The model under review builds one solid part; all positions refer to its coordinate system, in mm. Face numbers are marked on the shaded views. A direction names the side the tool comes from. Coordinates: 2 decimals unless noted, no trailing zeros. Loops run counter-clockwise (first coordinate to the right, second up) from the corner with the lowest first, then second, coordinate; pieces in that order, holes last. Notation, with made-up numbers: (58, -12.5) - (116, -12.5) arc R25 ccw to (116, 10.5) - close; hole circle Ø4 at (70, 10.25). An arc over 180 degrees is marked (long way). Use a Markdown table: item, result. Add a question column.
1) Clearance check with flat-ended pins moving along their axes: pin 1 (6 mm diameter, centred on x = 11, y = 0, fed in from +Z); pin 2 (5 mm diameter, centred on x = 15.5, y = 32.5, fed in from +Z); pin 3 (3 mm diameter, centred on y = 5.5, z = 37.5, fed in from +X). State where each tip first meets the part, or that it passes through.
2) For the marked faces 1, 2, 3 and 4, list the 3-axis set-ups (+Z, -Z, +X, -X, +Y, -Y) from which the entire face can be reached by the end or side of a thin tool; tool diameter is ignored.
3) Add section C-C, the plane x = 16.5. Give the boundary of the cut face in (y, z), and give its area (3 significant figures).
4) Add section D-D, the plane y = 11. Give the boundary of the cut face in (x, z).
5) Add section B-B, the plane y = 2. Give the boundary of the cut face in (x, z), and give its area (3 significant figures).
6) To check wall thickness, follow L1, parallel to X at y = 16.5, z = 23; L2, parallel to Z at x = 18.5, y = -7.5; L3, parallel to Y at x = 28, z = 47. State the ranges of each line that lie inside material, in increasing order. Write a range as [from, to].
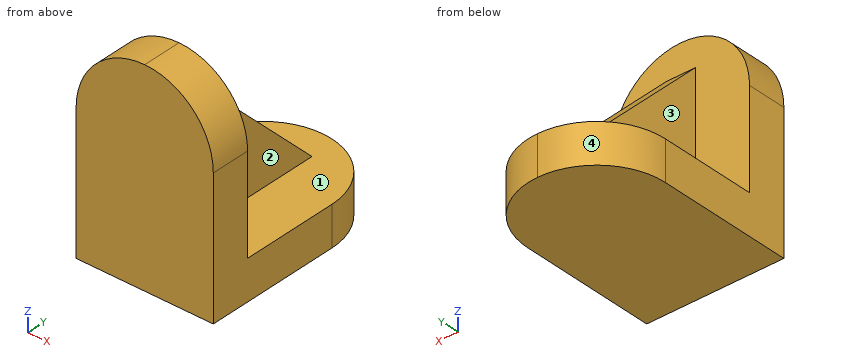
```python
from build123d import *

# Parameters (mm, degrees)
F1_DEPTH = 38
F2_R     = 18.99999
F3_R     = 18.99999
F6_DEPTH = 8


# Not quite as in the source:
# - a fillet or chamfer is up to 0.001 mm smaller than in the source, because OpenCascade refuses the exact size


with BuildPart() as f1:
    # F0 (on Right) → F1 (new body)
    with BuildSketch(Plane.YZ):
        Polygon((-14.4942225739, 53.3158381923), (-14.4942225739, -3.6841618077), (42.5057774261, -3.6841618077), (42.5057774261, 7.3158381923), (-3.4942225739, 7.3158381923), (-3.4942225739, 53.3158381923), align=None)
    extrude(amount=F1_DEPTH)

    # F2 (radius 19 in the source; OpenCascade refuses exactly that, so slightly less here)
    f2_edges = [f1.edges().sort_by_distance(p)[0] for p in [
        (38, -8.994223, 53.315838),
        (0, -8.994223, 53.315838),
    ]]
    fillet(f2_edges, radius=F2_R)

    # F3 (radius 19 in the source; OpenCascade refuses exactly that, so slightly less here)
    f3_edges = [f1.edges().sort_by_distance(p)[0] for p in [
        (38, 42.505777, 1.815838),
        (0, 42.505777, 1.815838),
    ]]
    fillet(f3_edges, radius=F3_R)

    # F5 (on offset) → F6 (join)
    with BuildSketch(Plane.YZ.offset(15)):
        Polygon((34.5057774261, 7.3158381923), (-3.4942225739, 45.3158381923), (-3.4942225739, 7.3158381923), align=None)
    extrude(amount=F6_DEPTH)


solid = f1.part
```
From the geometry:
| question | item | result |
|---|---|---|
| 1 | pin 1 | stops at z = 7.32 |
| 1 | pin 2 | stops at z = 11.82 |
| 1 | pin 3 | stops at x = 23 |
| 2 | face 1 | +Z, +X, +Y |
| 2 | face 2 | +Z, +X, +Y |
| 2 | face 3 | +Z, -X, +Y |
| 2 | face 4 | +Z, -Z, -X, +Y |
| 3 | outline | (-14.49, -3.68) - (42.34, -3.68) - (42.34, 7.32) - (34.51, 7.32) - (-3.49, 45.32) - (-3.49, 53.15) - (-14.49, 53.15) - close |
| 3 | area | 1,850 mm^2 |
| 4 | outline | (0, -3.68) - (38, -3.68) - (38, 7.32) - (23, 7.32) - (23, 30.82) - (15, 30.82) - (15, 7.32) - (0, 7.32) - close |
| 5 | outline | (0, -3.68) - (38, -3.68) - (38, 7.32) - (23, 7.32) - (23, 39.82) - (15, 39.82) - (15, 7.32) - (0, 7.32) - close |
| 5 | area | 678 mm^2 |
| 6 | L1 | x = [15, 23] |
| 6 | L2 | z = [-3.68, 53.31] |
| 6 | L3 | y = [-14.49, -3.49] |
